Build history of the part. All positions in model axes, mm. A direction names the side the tool comes from. Round coordinates to 2 decimals unless told otherwise and drop trailing zeros. Write each loop counter-clockwise with the first axis right and the second up, starting at its lowest first coordinate (ties: lowest second). Pieces come first, ordered by that corner, then holes.
Item 1: Band-saw the part on C-C, the plane z = 68.5. Write the cut outline in (x, y) (3 decimals).
Item 2: Band-saw the part on D-D, the plane z = 114.5. Write the cut outline in (x, y) (3 decimals).
Item 3: Drop flat-ended pins along their axis: pin 1 Ø8 at (y, z) = (-6.5, 112.5) entering from +X; pin 2 Ø8 at (y, z) = (131.5, 18.5) entering from +X; pin 3 Ø10 at (x, z) = (473.5, 109.5) entering from -Y. Give the stop position or say it passes through.
Item 4: Wall check: probe 1 along X at (y, z) = (304, 52); probe 2 along Y at (x, z) = (184, 60) (3 decimals); probe 3 along X at (y, z) = (532, 97). Give the ranges that are in metal, low to high.
Item 5: Band-saw the part on A-A, the plane x = 381. Write the cut outline in (y, z) (3 decimals), then the cut area to 3 significant figures.
Item 6: Band-saw the part on B-B, the plane y = 34. Write the cut outline in (x, z), then the cut area to 3 significant figures.
Item 7: Mould opens along X. For faces 1 (the cylindrical face through (-73.496, 628.627, 63.944)), 2 (the flat face through (351, 555.625, 63)), 3 (the flat face through (793.75, 273, 63)), 4 (the cylindrical face through (361.29, -73.5, 117.45)) say: +X half, -X half, draft (parallel to the pull), parting line (faces both ways), or undercut.
Item 8: 3-axis set-ups, long thin cutter, end or side, ignore diameter. For faces 5 (the flat face through (354, 571, 127)), 6 (the flat face through (0, 274, 63)): which of +Z, -Z, +X, -X, +Y, -Y reach the whole face in a straight line?
```python
from build123d import *

# Parameters (mm, degrees)
SKETCH1_W           = 876.3
SKETCH1_H           = 720.725
SKETCH1_W_2         = 711.2
SKETCH1_H_2         = 555.625
BOSS_EXTRUDE1_DEPTH = 127
FILLET1_R           = 31.75


with BuildPart() as part:
    # Sketch1 → Boss-Extrude1 (new body)
    with BuildSketch(Plane.XY):
        with Locations((355.6, 277.8125)):
            Rectangle(SKETCH1_W, SKETCH1_H)
        with Locations((355.6, 277.8125)):
            Rectangle(SKETCH1_W_2, SKETCH1_H_2, mode=Mode.SUBTRACT)
    extrude(amount=BOSS_EXTRUDE1_DEPTH)

    # Fillet1
    fillet1_edges = [part.edges().sort_by_distance(p)[0] for p in [
        (355.6, 638.175, 127),
        (355.6, -82.55, 0),
        (-82.55, 277.8125, 0),
        (355.6, 638.175, 0),
        (793.75, 277.8125, 0),
        (-82.55, 277.8125, 127),
        (793.75, -82.55, 63.5),
        (-82.55, -82.55, 63.5),
        (-82.55, 638.175, 63.5),
        (793.75, 638.175, 63.5),
        (355.6, -82.55, 127),
        (793.75, 277.8125, 127),
    ]]
    fillet(fillet1_edges, radius=FILLET1_R)


solid = part.part
```
Results:
1. outline: (-82.55, -50.8) arc R31.75 ccw to (-50.8, -82.55) - (762, -82.55) arc R31.75 ccw to (793.75, -50.8) - (793.75, 606.425) arc R31.75 ccw to (762, 638.175) - (-50.8, 638.175) arc R31.75 ccw to (-82.55, 606.425) - close; hole (0, 0) - (711.2, 0) - (711.2, 555.625) - (0, 555.625) - close
2. outline: (-76.049, -50.8) arc R25.249 ccw to (-50.8, -76.049) - (762, -76.049) arc R25.249 ccw to (787.249, -50.8) - (787.249, 606.425) arc R25.249 ccw to (762, 631.674) - (-50.8, 631.674) arc R25.249 ccw to (-76.049, 606.425) - close; hole (0, 0) - (711.2, 0) - (711.2, 555.625) - (0, 555.625) - close
3. pin 1: stops at x = 790.85
3. pin 2: stops at x = 792.37
3. pin 3: stops at y = -81.17
4. probe 1: x = -82.55 to 0, 711.2 to 793.75
4. probe 2: y = -82.55 to 0, 555.625 to 638.175
4. probe 3: x = -82.5 to 0, 711.2 to 793.7
5. outline: (-82.55, 31.75) arc R31.75 ccw to (-50.8, 0) - (0, 0) - (0, 127) - (-50.8, 127) arc R31.75 ccw to (-82.55, 95.25) - close; (555.625, 0) - (606.425, 0) arc R31.75 ccw to (638.175, 31.75) - (638.175, 95.25) arc R31.75 ccw to (606.425, 127) - (555.625, 127) - close
5. area: 20,100 mm2
6. outline: (-82.55, 31.75) arc R31.75 ccw to (-50.8, 0) - (0, 0) - (0, 127) - (-50.8, 127) arc R31.75 ccw to (-82.55, 95.25) - close; (711.2, 0) - (762, 0) arc R31.75 ccw to (793.75, 31.75) - (793.75, 95.25) arc R31.75 ccw to (762, 127) - (711.2, 127) - close
6. area: 20,100 mm2
7. face 1: -X half
7. face 2: undercut
7. face 3: +X half
7. face 4: draft
8. face 5: +Z, +X, -X, +Y, -Y
8. face 6: +Z, -Z
